Part model, mm, in its own coordinate system. A direction names the side the tool comes from. Coordinates: 2 decimals unless noted, no trailing zeros. Use a Markdown table: item, result. Add a question column.
1) Wall check: probe 1 along Z at (x, y) = (-9.75, 1.25); probe 2 along X at (y, z) = (1, 9); probe 3 along Z at (x, y) = (4, 2). Give the ranges that are in metal, low to high. Write a range as from..to.
2) Pin check, flat tips, straight feed: pin 1 Ø3 at (x, z) = (-8, 10.5) entering from +Y; pin 2 Ø5 at (x, z) = (0.5, -3.5) entering from -Y; pin 3 Ø1 at (y, z) = (1.5, 3) entering from -X; pin 4 Ø6 at (x, z) = (0.5, -1.5) entering from +Y. Stop position of each tip, or through.
3) Tool access for faces 1 (the cylindrical face through (-8.133, 2.958, -5.473)), 2 (the flat face through (6, -1.588, 6)): list every direction of +Z, -Z, +X, -X, +Y, -Y with a clear straight run to the whole face (end or side of a thin tool).
4) Pull direction X, two halves, no side cores. Call faces 3 (the cylindrical face through (10.418, -1.185, 7.988)), 4 (the flat face through (2, 0, -11)), 5 (the cylindrical face through (5.42, 2.96, 8.17)), 6 (the flat face through (5, 6, 0)): released by +X, released by -X, zero draft, split by the parting line, or undercut.
from build123d import *

# Parameters (mm, degrees)
SKETCH1_R           = 12.732395445
BOSS_EXTRUDE1_DEPTH = 6
CUT_EXTRUDE1_DEPTH  = 6
CIRPATTERN1_COUNT   = 16
SKETCH4_R           = 7.9375
SKETCH4_R_2         = 4.7625
CUT_EXTRUDE4_DEPTH  = 5
SKETCH4_5_R         = 4.7625
CUT_EXTRUDE5_DEPTH  = 8.5875


with BuildPart() as part:
    # Sketch1 → Boss-Extrude1 (new body)
    with BuildSketch(Plane(origin=(0, 0, 0), x_dir=(1, 0, 0), z_dir=(0, 1, 0))):
        Circle(SKETCH1_R)
    extrude(amount=BOSS_EXTRUDE1_DEPTH)

    # Sketch3 → Cut-Extrude1 (cut)
    with BuildSketch(Plane(origin=(0, 0, 0), x_dir=(1, 0, 0), z_dir=(0, 1, 0))):
        with BuildLine():
            Line((5.255160224, 12.687079084), (4.539542206, 10.959424358))
            ThreePointArc((4.539542206, 10.959424358), (4.387777638, 11.021063156), (4.235176409, 11.080600457))
            ThreePointArc((4.235176409, 11.080600457), (3.875932689, 11.056534938), (3.660923238, 10.767733734))
            ThreePointArc((3.660923238, 10.767733734), (1.912352484, 9.614045165), (0.738381256, 11.349063479))
            ThreePointArc((0.738381256, 11.349063479), (0.65025786, 11.698161555), (0.327569416, 11.857871815))
            ThreePointArc((0.327569416, 11.857871815), (0.163800325, 11.861264483), (0, 11.862395445))
            Line((0, 11.862395445), (0, 13.732395445))
            ThreePointArc((0, 13.732395445), (2.67905745, 13.468531317), (5.255160224, 12.687079084))
        make_face()
    cut_extrude1 = extrude(amount=CUT_EXTRUDE1_DEPTH, mode=Mode.SUBTRACT)

    # CirPattern1: Cut-Extrude1 ×16 about axis
    cirpattern1_axis = Axis((0, 0, 0), (0, 1, 0))
    for i in range(1, CIRPATTERN1_COUNT):
        add(cut_extrude1.rotate(cirpattern1_axis, i * 360 / CIRPATTERN1_COUNT), mode=Mode.SUBTRACT)

    # Sketch5 → Revolve1 (revolve)
    with BuildSketch(Plane.XY):
        Polygon((0, 0), (0, -1.5875), (-13.127871815, -1.5875), (-13.127871815, -0.79375), (-11.857871815, 0), align=None)
    revolve(axis=Axis((0, 0, 0), (0, -1, 0)))

    # Sketch4 → Cut-Extrude4 (cut)
    with BuildSketch(Plane.XZ.offset(1.5875)):
        Circle(SKETCH4_R)
        Circle(SKETCH4_R_2, mode=Mode.SUBTRACT)
    extrude(amount=-CUT_EXTRUDE4_DEPTH, mode=Mode.SUBTRACT)

    # Sketch4<5> → Cut-Extrude5 (cut, through all)
    with BuildSketch(Plane.XZ.offset(1.5875)):
        Circle(SKETCH4_5_R)
    extrude(amount=-CUT_EXTRUDE5_DEPTH, mode=Mode.SUBTRACT)


solid = part.part
Entries:
| question | item | result |
|---|---|---|
| 1 | probe 1 | -4.83..-2.88, -1.52..1.52, 2.88..4.83 |
| 1 | probe 2 | -4.84..4.84 |
| 1 | probe 3 | -11.1..-6.86, 6.86..11.1 |
| 2 | pin 1 | y = 0 |
| 2 | pin 2 | y = 3.41 |
| 2 | pin 3 | x = -10.34 |
| 2 | pin 4 | through |
| 3 | face 1 | +Y |
| 3 | face 2 | +Z, -Z, +X, -X, -Y |
| 4 | face 3 | split by the parting line |
| 4 | face 4 | undercut |
| 4 | face 5 | undercut |
| 4 | face 6 | zero draft |
